from build123d import *

# Parameters (mm, degrees)
BOSS_EXTRUDE1_DEPTH     = 114.3
SKETCH2_R               = 3.3274
CUT_EXTRUDE1_DEPTH      = 133.134940496
CUT_EXTRUDE2_REACH      = 128.523
CUT_EXTRUDE2_END_RADIUS = 12.7
SKETCH3_R               = 6.35


with BuildPart() as part:
    # Sketch1 → Boss-Extrude1 (new body)
    with BuildSketch(Plane.XY):
        with BuildLine():
            Line((4.010170085, 26.049749551), (11.717651581, 12.7))
            Line((11.717651581, 12.7), (19.05, 12.7))
            Line((19.05, 12.7), (19.05, 76.2))
            Line((19.05, 76.2), (-19.05, 76.2))
            Line((-19.05, 76.2), (-19.05, 12.7))
            Line((-19.05, 12.7), (-11.717651581, 12.7))
            Line((-11.717651581, 12.7), (-4.010170085, 26.049749551))
            ThreePointArc((-4.010170085, 26.049749551), (0, 50.8), (4.010170085, 26.049749551))
        make_face()
    extrude(amount=BOSS_EXTRUDE1_DEPTH)

    # Sketch2 → Cut-Extrude1 (cut, through all)
    with BuildSketch(Plane(origin=(0, 76.2, 0), x_dir=(1, 0, 0), z_dir=(0, 1, 0))):
        with Locations(Location((0, -19.05, 0), (0, 0, 270))):
            Circle(SKETCH2_R)
        with Locations(Location((0, -57.15, 0), (0, 0, 270))):
            Circle(SKETCH2_R)
        with Locations(Location((0, -95.25, 0), (0, 0, 270))):
            Circle(SKETCH2_R)
    extrude(amount=-CUT_EXTRUDE1_DEPTH, mode=Mode.SUBTRACT)

    # Cut-Extrude2: up to this cylinder (the profile starts outside it)
    cut_extrude2_end = Plane(origin=(0, 38.1, 57.15), z_dir=(0, 0, -1)) * Cylinder(CUT_EXTRUDE2_END_RADIUS, 359.646, mode=Mode.PRIVATE)
    # Sketch3 → Cut-Extrude2 (cut, up to the surface)
    with BuildSketch(Plane(origin=(0, 63.5, 0), x_dir=(1, 0, 0), z_dir=(0, 1, 0)), mode=Mode.PRIVATE) as cut_extrude2_sk1:
        with Locations(Location((0, -19.05, 0), (0, 0, 270))):
            Circle(SKETCH3_R)
    cut_extrude2_tool1 = extrude(cut_extrude2_sk1.sketch, amount=-CUT_EXTRUDE2_REACH, mode=Mode.PRIVATE) - cut_extrude2_end
    add(cut_extrude2_tool1.solids().sort_by_distance((0, 63.5, 19.05))[0], mode=Mode.SUBTRACT)
    # Sketch3 → Cut-Extrude2 (cut, up to the surface)
    with BuildSketch(Plane(origin=(0, 63.5, 0), x_dir=(1, 0, 0), z_dir=(0, 1, 0)), mode=Mode.PRIVATE) as cut_extrude2_sk2:
        with Locations(Location((0, -57.15, 0), (0, 0, 270))):
            Circle(SKETCH3_R)
    cut_extrude2_tool2 = extrude(cut_extrude2_sk2.sketch, amount=-CUT_EXTRUDE2_REACH, mode=Mode.PRIVATE) - cut_extrude2_end
    add(cut_extrude2_tool2.solids().sort_by_distance((0, 63.5, 57.15))[0], mode=Mode.SUBTRACT)
    # Sketch3 → Cut-Extrude2 (cut, up to the surface)
    with BuildSketch(Plane(origin=(0, 63.5, 0), x_dir=(1, 0, 0), z_dir=(0, 1, 0)), mode=Mode.PRIVATE) as cut_extrude2_sk3:
        with Locations(Location((0, -95.25, 0), (0, 0, 270))):
            Circle(SKETCH3_R)
    cut_extrude2_tool3 = extrude(cut_extrude2_sk3.sketch, amount=-CUT_EXTRUDE2_REACH, mode=Mode.PRIVATE) - cut_extrude2_end
    add(cut_extrude2_tool3.solids().sort_by_distance((0, 63.5, 95.25))[0], mode=Mode.SUBTRACT)


solid = part.part
Source: CAD feature listing. Evaluate the final solid. Frame: model axes, mm. A direction names the side the tool comes from. Round coordinates to 2 decimals unless told otherwise and drop trailing zeros. Order: outer loops, then holes, each group sorted by start corner. A loop starts at its lowest first (then second) coordinate and runs counter-clockwise, first axis right, second up. Notation, with made-up numbers: (77.5, -12) -> (133.5, -12) arc R16 ccw to (133.5, 2) -> close; hole circle Ø5 at (36, -2.75). An arc over 180 degrees is marked (long way). Answer as CSV lines item,"result".
Item 1: Section C-C, the plane x = -9.5. Return loops of the section in (y, z), plus the area to 3 significant figures.
A:
outline,"(16.54, 0) -> (29.67, 0) -> (29.67, 114.3) -> (16.54, 114.3) -> close; (46.53, 0) -> (76.2, 0) -> (76.2, 114.3) -> (46.53, 114.3) -> close"
area,"4,890 mm²"
Item 2: Pin query (flat end, axial travel): pin 1 Ø5 at (x, z) = (-9, 73.5) entering from -Y; pin 2 Ø4 at (x, z) = (3, 16) entering from -Y; pin 3 Ø7.5 at (x, z) = (0, 95.25) entering from -Y. Return the tip coordinate at first contact, or that it passes through.
A:
pin 1,"y = 13.08"
pin 2,"y = 24.34"
pin 3,"y = 63.5"
Item 3: Line query: L1, parallel to Z at x = 0, y = 52; L2, parallel to X at y = 59, z = 19.05; L3, parallel to X at y = 67.25, z = 95.25. Output: solid intervals per line, ascending.
A:
L1,"0 to 12.7, 25.4 to 50.8, 63.5 to 88.9, 101.6 to 114.3"
L2,"-19.05 to -6.35, 6.35 to 19.05"
L3,"-19.05 to -3.33, 3.33 to 19.05"
Item 4: Reachability of faces 5 (the face through (-7.92, 19.28, 56.35)), 6 (the face through (1.907, 56.4, 101.307)), 7 (the face through (0.146, 69.939, 53.826)) from +Z, -Z, +X, -X, +Y, -Y: full face, straight path, thin tool, end or side. Return the list, or none.
A:
face 5,"+Z, -Z, -Y"
face 6,"none"
face 7,"+Y, -Y"
Item 5: Section B-B, the plane y = 54. Return loops of the section in (x, z).
A:
outline,"(-19.05, 0) -> (19.05, 0) -> (19.05, 114.3) -> (-19.05, 114.3) -> close; hole circle Ø12.7 at (0, 19.05); hole circle Ø12.7 at (0, 57.15); hole circle Ø12.7 at (0, 95.25)"
Item 6: Section D-D, the plane z = 73. Return loops of the section in (x, y).
A:
outline,"(-19.05, 12.7) -> (-11.72, 12.7) -> (-4.01, 26.05) arc R12.7 cw (long way) to (4.01, 26.05) -> (11.72, 12.7) -> (19.05, 12.7) -> (19.05, 76.2) -> (-19.05, 76.2) -> close"
Item 7: Pull-direction query (Y, two-part tool) for faces 1 (the face through (-15, 12.7, 56)), 2 (the face through (1.907, 56.4, 63.207)), 3 (the face through (0, 52, 114.3)), 4 (the face through (-3, 63.5, 22)); classes: pulls with the +Y half, pulls with the -Y half, needs draft (parallel to the pull), parting line crosses it, or undercut.
A:
face 1,"pulls with the -Y half"
face 2,"undercut"
face 3,"needs draft"
face 4,"undercut"
Item 8: Section A-A, the plane z = 19.05. Return loops of the section in (x, y).
A:
outline,"(-19.05, 12.7) -> (-11.72, 12.7) -> (-4.01, 26.05) arc R12.7 cw to (-6.35, 49.1) -> (-6.35, 63.5) -> (-3.33, 63.5) -> (-3.33, 76.2) -> (-19.05, 76.2) -> close; (3.33, 63.5) -> (6.35, 63.5) -> (6.35, 49.1) arc R12.7 cw to (4.01, 26.05) -> (11.72, 12.7) -> (19.05, 12.7) -> (19.05, 76.2) -> (3.33, 76.2) -> close"
